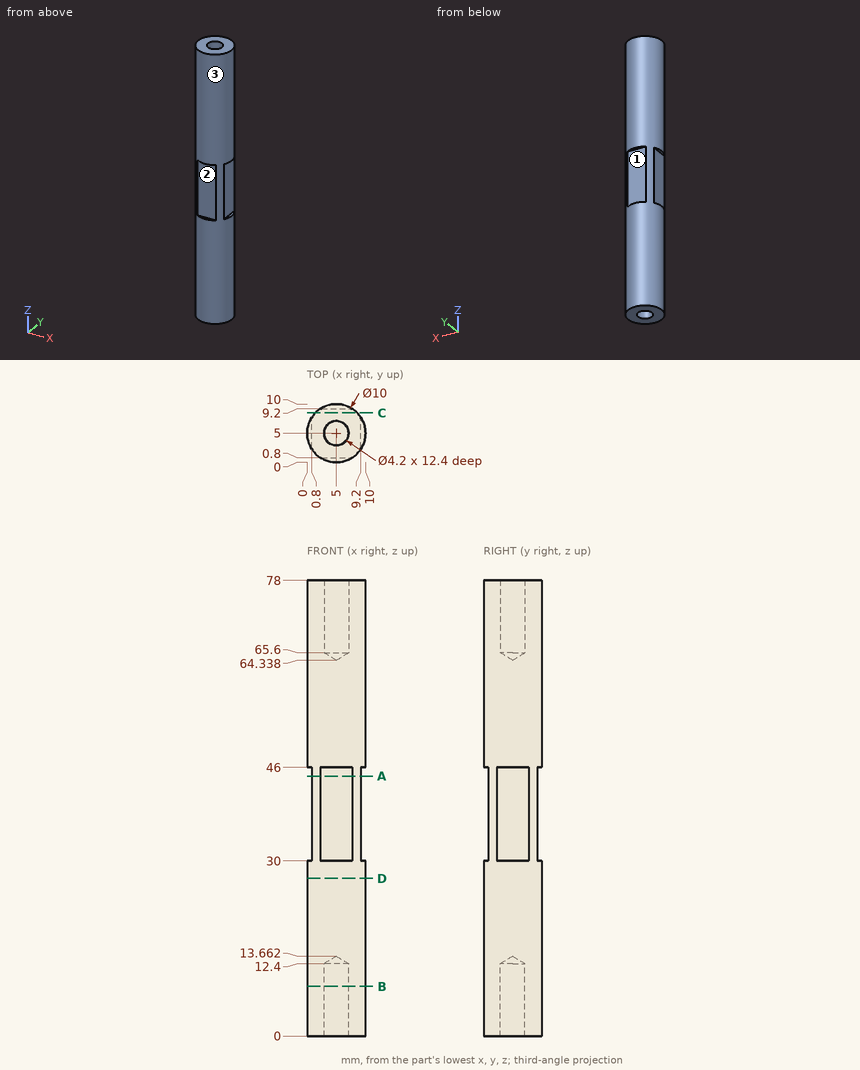
Job drawing, mm, ordinate dimensions from the low corner. One solid piece. Coordinates: 2 decimals unless noted, no trailing zeros. Loops run counter-clockwise (first coordinate to the right, second up) from the corner with the lowest first, then second, coordinate; pieces in that order, holes last. Notation, with made-up numbers: (45.25, -24) - (82.25, -24) arc R12 ccw to (82.25, -10) - close; hole circle Ø8 at (3.25, -15). An arc over 180 degrees is marked (long way). Write item = value, one per line. Start each with the question number.
Q1. Pull direction Z, two halves, no side cores. Call the marked faces 1, 2 and 3: pulls with the +Z half, pulls with the -Z half, needs draft (parallel to the pull), parting line crosses it, or undercut.
Q2. Cut at C-C, the plane y = 8.5. List the corners of the cut face in (x, z), then the cut area to 3 significant figures.
Q3. Drill centre lines: L1, parallel to Y at x = 5, z = 75.5; L2, parallel to Y at x = 5.75, z = 42.5. Where is each one in solid material? Low to high.
Q4. Cut at B-B, the plane z = 8.5. List the corners of the cut face in (x, y).
Q5. Cut at D-D, the plane z = 27. List the corners of the cut face in (x, y).
Q6. Cut at A-A, the plane z = 44.5. List the corners of the cut face in (x, y).
Q7. Flat gauge pins, fed straight in: pin 1 Ø1.5 at (x, z) = (1, 13.5) entering from -Y; pin 2 Ø3.5 at (x, y) = (5, 5) entering from -Z; pin 3 Ø2.5 at (x, y) = (5, 5) entering from +Z. Where does each tip first touch, or does it go through?
Computed:
q1.face_1 = undercut
q1.face_2 = undercut
q1.face_3 = needs draft
q2.outline = (1.43, 0) - (8.57, 0) - (8.57, 78) - (1.43, 78) - close
q2.area = 557 mm²
q3.L1 = 0 to 2.9, 7.1 to 10
q3.L2 = 0.8 to 9.2
q4.outline = circle Ø10 at (5, 5); hole circle Ø4.2 at (5, 5)
q5.outline = circle Ø10 at (5, 5)
q6.outline = (0.8, 2.29) arc R5 ccw to (2.29, 0.8) - (7.71, 0.8) arc R5 ccw to (9.2, 2.29) - (9.2, 7.71) arc R5 ccw to (7.71, 9.2) - (2.29, 9.2) arc R5 ccw to (0.8, 7.71) - close
q7.pin_1 = 1.2
q7.pin_2 = 12.61
q7.pin_3 = 65.09
